Build history of the part. All positions in model axes, mm. Face numbers are marked on the shaded views. A direction names the side the tool comes from. Give positions to 0.01 mm unless a question says otherwise; leave off trailing zeros. Loops run counter-clockwise (first coordinate to the right, second up) from the corner with the lowest first, then second, coordinate; pieces in that order, holes last.
1) Wall check: line 1 (Y direction, x = 38, z = 5.8); line 2 (Z direction, x = 28.5, y = 67); line 3 (Z direction, x = -13, y = 23). Give the ranges that are in metal, low to high.
2) Flat gauge pins, fed straight in: P1, Ø1, axis at x = 73, y = 62, coming from the +Z side; P2, Ø8.5, axis at x = 25, z = 78.88, coming from the +Y side; P3, Ø4.5, axis at x = 18.5, z = 79, coming from the -Y side. Where does each tip first touch, or does it go through?
3) Band-saw the part on B-B on y = 77. List the corners of the cut face in (x, z), then the cut area to 3 significant figures.
4) Band-saw the part on C-C on x = 13.5. List the corners of the cut face in (y, z), then the cut area to 3 significant figures.
5) Band-saw the part on D-D on y = 55. List the corners of the cut face in (x, z), then the cut area to 3 significant figures.
6) Two-plate mould, pull along Y, no slides. Class the marked faces 1, 2 and 3: +Y half, -Y half, draft (parallel to the pull), parting line (faces both ways), or undercut.
7) Band-saw the part on A-A on x = 25. List the corners of the cut face in (y, z).
8) 3-axis set-ups, long thin cutter, end or side, ignore diameter. For the marked faces 4 and 5: which of +Z, -Z, +X, -X, +Y, -Y reach the whole face in a straight line?
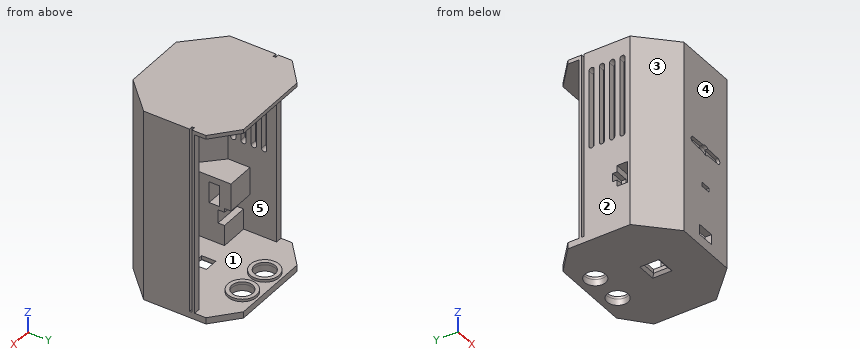
```python
from build123d import *

# Parameters (mm, degrees)
BOSS_EXTRUDE2_DEPTH  = 150
CUT_EXTRUDE2_DEPTH   = 145
CUT_EXTRUDE4_DEPTH   = 145
BOSS_EXTRUDE3_DEPTH  = 90
SKETCH10_W           = 14
SKETCH10_H           = 8
SKETCH10_W_2         = 8.5
SKETCH10_H_2         = 3.2
CUT_EXTRUDE5_DEPTH   = 189.01595677
SKETCH11_W           = 11
SKETCH11_H           = 11
CUT_EXTRUDE6_DEPTH   = 187.413518823
SKETCH12_R           = 11.15
SKETCH12_R_2         = 8.15
BOSS_EXTRUDE4_DEPTH  = 2
SKETCH13_R           = 8.15
CUT_EXTRUDE7_DEPTH   = 187.413518823
CHAMFER1_SIZE        = 2
CUT_EXTRUDE8_REACH   = 166.515
SKETCH14_W           = 45.857864376
SKETCH14_H           = 8
BOSS_EXTRUDE5_REACH  = 179.757
SKETCH15_W           = 22.071067812
SKETCH15_H           = 16.5
BOSS_EXTRUDE6_REACH  = 179.757
SKETCH16_W           = 22.071067812
SKETCH16_H           = 16.5
BOSS_EXTRUDE7_DEPTH  = 22.071067812
BOSS_EXTRUDE9_DEPTH  = 3
SKETCH19_W           = 1
SKETCH19_H           = 2
BOSS_EXTRUDE10_DEPTH = 142
CUT_EXTRUDE9_DEPTH   = 151.203195705
SKETCH21_W           = 16.5
SKETCH21_H           = 8
CUT_EXTRUDE10_DEPTH  = 200.060292374
SKETCH22_W           = 6.5
SKETCH22_H           = 3.5
CUT_EXTRUDE11_DEPTH  = 10
CUT_EXTRUDE13_DEPTH  = 5
CUT_EXTRUDE15_DEPTH  = 2.5
SKETCH28_R           = 3.8
CUT_EXTRUDE16_DEPTH  = 190.15932438
BOSS_EXTRUDE11_DEPTH = 13


with BuildPart() as part:
    # Sketch1 → Boss-Extrude2 (new body)
    with BuildSketch(Plane.XY):
        Polygon((0, 0), (50, 0), (75, 25), (75, 73.483551981), (56, 90), (-6, 90), (-25, 73.483551981), (-25, 25), align=None)
    extrude(amount=BOSS_EXTRUDE2_DEPTH)

    # Sketch3 → Cut-Extrude2 (cut)
    with BuildSketch(Plane.XY.offset(150)):
        Polygon((-4.130576603, 85), (-20, 71.204920704), (-20, 27.071067812), (2.071067812, 5), (47.928932188, 5), (70, 27.071067812), (70, 71.204920704), (54.130576603, 85), align=None)
    extrude(amount=-CUT_EXTRUDE2_DEPTH, mode=Mode.SUBTRACT)

    # Sketch8 → Cut-Extrude4 (cut)
    with BuildSketch(Plane.XY.offset(150)):
        Polygon((-6, 90), (-25, 73.483551981), (-25, 60.75095761), (-22, 60.75095761), (-22, 62.75095761), (-24, 62.75095761), (-24, 64.75095761), (-20, 64.75095761), (-20, 71.204920704), (-4.130576603, 85), (54.130576603, 85), (70, 71.204920704), (70, 64.75095761), (74, 64.75095761), (74, 62.75095761), (72, 62.75095761), (72, 60.75095761), (75, 60.75095761), (75, 73.483551981), (56, 90), align=None)
    extrude(amount=-CUT_EXTRUDE4_DEPTH, mode=Mode.SUBTRACT)

    # Sketch9 → Boss-Extrude3 (add)
    with BuildSketch(Plane.ZY.offset(-70)):
        Polygon((21, 34.071067812), (31.5, 34.071067812), (31.5, 39.071067812), (34.5, 39.071067812), (34.5, 31.071067812), (18, 31.071067812), (18, 39.071067812), (21, 39.071067812), align=None)
    extrude(amount=BOSS_EXTRUDE3_DEPTH)

    # Sketch10 → Cut-Extrude5 (cut, through all)
    with BuildSketch(Plane(origin=(0, 5, 0), x_dir=(1, 0, 0), z_dir=(0, 1, 0))):
        with Locations((25, -12)):
            Rectangle(SKETCH10_W, SKETCH10_H)
        with Locations((25, -49.625084235)):
            Rectangle(SKETCH10_W_2, SKETCH10_H_2)
    extrude(amount=-CUT_EXTRUDE5_DEPTH, mode=Mode.SUBTRACT)

    # Sketch11 → Cut-Extrude6 (cut, through all)
    with BuildSketch(Plane.XY.offset(5)):
        with Locations((25, 38.5)):
            Rectangle(SKETCH11_W, SKETCH11_H)
    extrude(amount=-CUT_EXTRUDE6_DEPTH, mode=Mode.SUBTRACT)

    # Sketch12 → Boss-Extrude4 (add)
    # profile 1 of 2: a face of its own
    with BuildSketch(Plane.XY.offset(5)):
        with Locations(Location((12, 77, 0), (0, 0, 180))):
            Circle(SKETCH12_R)
        with Locations((12, 77)):
            Circle(SKETCH12_R_2, mode=Mode.SUBTRACT)
    # profile 2 of 2: a face of its own
    with BuildSketch(Plane.XY.offset(5)):
        with Locations(Location((38, 77, 0), (0, 0, 180))):
            Circle(SKETCH12_R)
        with Locations((38, 77)):
            Circle(SKETCH12_R_2, mode=Mode.SUBTRACT)
    extrude(amount=BOSS_EXTRUDE4_DEPTH)

    # Sketch13 → Cut-Extrude7 (cut, through all)
    with BuildSketch(Plane.XY.offset(5)):
        with Locations((12, 77)):
            Circle(SKETCH13_R)
        with Locations((38, 77)):
            Circle(SKETCH13_R)
    extrude(amount=-CUT_EXTRUDE7_DEPTH, mode=Mode.SUBTRACT)

    # Chamfer1
    chamfer1_edges = [part.edges().sort_by_distance(p)[0] for p in [
        (19.5, 38.5, 0),
        (25, 44, 0),
        (30.5, 38.5, 0),
        (25, 33, 0),
    ]]
    chamfer(chamfer1_edges, length=CHAMFER1_SIZE)

    # Cut-Extrude8: up to this face of the body (flat: up to its plane)
    cut_extrude8_end = Plane(part.part.faces().sort_by_distance((25, 35.071067812, 18))[0])
    # Sketch14 → Cut-Extrude8 (cut, up to the picked face)
    with BuildSketch(Plane.XY.offset(34.5), mode=Mode.PRIVATE) as cut_extrude8_sk1:
        with Locations((25, 35.071067812)):
            Rectangle(SKETCH14_W, SKETCH14_H)
    cut_extrude8_tool1 = split(extrude(cut_extrude8_sk1.sketch, amount=-CUT_EXTRUDE8_REACH, mode=Mode.PRIVATE), bisect_by=cut_extrude8_end, keep=Keep.BOTH, mode=Mode.PRIVATE)
    add(cut_extrude8_tool1.solids().sort_by(Axis((25, 35.071068, 34.5), (0, 0, -1)))[0], mode=Mode.SUBTRACT)

    # Boss-Extrude5: up to this plane
    boss_extrude5_end = Plane(origin=(47.928932188, 5, -120.415945788), z_dir=(0.7071067811865476, -0.7071067811865475, 0))
    # Sketch15 → Boss-Extrude5 (add, up to the surface)
    with BuildSketch(Plane.XZ.offset(-31.071067812), mode=Mode.PRIVATE) as boss_extrude5_sk1:
        with Locations((58.964466094, 26.25)):
            Rectangle(SKETCH15_W, SKETCH15_H)
    boss_extrude5_tool1 = split(extrude(boss_extrude5_sk1.sketch, amount=BOSS_EXTRUDE5_REACH, mode=Mode.PRIVATE), bisect_by=boss_extrude5_end, keep=Keep.BOTH, mode=Mode.PRIVATE)
    add(boss_extrude5_tool1.solids().sort_by_distance((58.964466, 31.071068, 26.25))[0])

    # Boss-Extrude6: up to this plane
    boss_extrude6_end = Plane(origin=(-20, 27.071067812, -120.415945788), z_dir=(-0.7071067811865475, -0.7071067811865476, 0))
    # Sketch16 → Boss-Extrude6 (add, up to the surface)
    with BuildSketch(Plane.XZ.offset(-31.071067812), mode=Mode.PRIVATE) as boss_extrude6_sk1:
        with Locations((-8.964466094, 26.25)):
            Rectangle(SKETCH16_W, SKETCH16_H)
    boss_extrude6_tool1 = split(extrude(boss_extrude6_sk1.sketch, amount=BOSS_EXTRUDE6_REACH, mode=Mode.PRIVATE), bisect_by=boss_extrude6_end, keep=Keep.BOTH, mode=Mode.PRIVATE)
    add(boss_extrude6_tool1.solids().sort_by_distance((-8.964466, 31.071068, 26.25))[0])

    # Sketch17 → Boss-Extrude7 (add)
    with BuildSketch(Plane(origin=(-20, 0, 0), x_dir=(0, 0, -1), z_dir=(1, 0, 0))):
        Polygon((-56, 27.071067812), (-51, 27.071067812), (-51, 35.071067812), (-34.5, 35.071067812), (-34.5, 39.071067812), (-34.5, 44.071067812), (-56, 44.071067812), align=None)
        Polygon((-34.5, 5), (-34.5, 27.071067812), (-51, 27.071067812), (-56, 27.071067812), (-56, 5), align=None)
    extrude(amount=BOSS_EXTRUDE7_DEPTH)

    # Sketch18 → Boss-Extrude9 (add)
    with BuildSketch(Plane.XY.offset(150)):
        Polygon((75, 62.75095761), (75, 73.483551981), (56, 90), (-6, 90), (-25, 73.483551981), (-25, 62.75095761), (-24, 62.75095761), (-24, 64.75095761), (-20, 64.75095761), (-20, 27.071067812), (2.071067812, 5), (47.928932188, 5), (70, 27.071067812), (70, 64.75095761), (74, 64.75095761), (74, 62.75095761), align=None)
    extrude(amount=-BOSS_EXTRUDE9_DEPTH)

    # Sketch19 → Boss-Extrude10 (add)
    with BuildSketch(Plane(origin=(0, 0, 147), x_dir=(-1, 0, 0), z_dir=(0, 0, -1))):
        with Locations((-74.5, 63.75095761)):
            Rectangle(SKETCH19_W, SKETCH19_H)
        with Locations((24.5, 63.75095761)):
            Rectangle(SKETCH19_W, SKETCH19_H)
    extrude(amount=BOSS_EXTRUDE10_DEPTH)

    # Sketch20 → Cut-Extrude9 (cut, through all)
    with BuildSketch(Plane.XY.offset(56)):
        Polygon((-5, 5), (-20, 20), (-20, 5), align=None)
    extrude(amount=-CUT_EXTRUDE9_DEPTH, mode=Mode.SUBTRACT)

    # Sketch21 → Cut-Extrude10 (cut, through all)
    with BuildSketch(Plane(origin=(-20, 0, 0), x_dir=(0, 0, -1), z_dir=(1, 0, 0))):
        with Locations((-42.75, 31.071067812)):
            Rectangle(SKETCH21_W, SKETCH21_H)
    extrude(amount=-CUT_EXTRUDE10_DEPTH, mode=Mode.SUBTRACT)

    # Sketch22 → Cut-Extrude11 (cut)
    with BuildSketch(Plane.ZY.offset(25)):
        with Locations((42.75, 36.821067812)):
            Rectangle(SKETCH22_W, SKETCH22_H)
    extrude(amount=-CUT_EXTRUDE11_DEPTH, mode=Mode.SUBTRACT)

    # Sketch23 → Cut-Extrude13 (cut)
    with BuildSketch(Plane.ZY.offset(25)):
        with BuildLine():
            Line((75, 29), (135, 29))
            ThreePointArc((135, 29), (137, 31), (135, 33))
            Line((135, 33), (75, 33))
            ThreePointArc((75, 33), (73, 31), (75, 29))
        make_face()
        with BuildLine():
            Line((135, 41), (75, 41))
            ThreePointArc((75, 41), (73, 39), (75, 37))
            Line((75, 37), (135, 37))
            ThreePointArc((135, 37), (137, 39), (135, 41))
        make_face()
        with BuildLine():
            Line((135, 49), (75, 49))
            ThreePointArc((75, 49), (73, 47), (75, 45))
            Line((75, 45), (135, 45))
            ThreePointArc((135, 45), (137, 47), (135, 49))
        make_face()
        with BuildLine():
            Line((135, 57), (75, 57))
            ThreePointArc((75, 57), (73, 55), (75, 53))
            Line((75, 53), (135, 53))
            ThreePointArc((135, 53), (137, 55), (135, 57))
        make_face()
    extrude(amount=-CUT_EXTRUDE13_DEPTH, mode=Mode.SUBTRACT)

    # Sketch27 → Cut-Extrude15 (cut)
    with BuildSketch(Plane.XZ):
        with BuildLine():
            Line((39.404762454, 81.167250077), (39.404762454, 81.166207685))
            ThreePointArc((39.404762454, 81.166207685), (41.672056129, 78.884218387), (39.404762454, 76.60222909))
            Line((39.404762454, 76.60222909), (39.404762454, 76.601183426))
            Line((39.404762454, 76.601183426), (27.659446006, 76.169652537))
            ThreePointArc((27.659446006, 76.169652537), (25.117179913, 75.085745409), (22.512932044, 76.010874907))
            Line((22.512932044, 76.010874907), (10.566254086, 76.601183426))
            ThreePointArc((10.566254086, 76.601183426), (8.393884355, 78.898098023), (10.595237546, 81.167250077))
            Line((10.595237546, 81.167250077), (22.340553994, 81.598223966))
            ThreePointArc((22.340553994, 81.598223966), (25, 82.683938251), (27.659446006, 81.598223966))
            Line((27.659446006, 81.598223966), (39.404762454, 81.167250077))
        make_face()
    extrude(amount=-CUT_EXTRUDE15_DEPTH, mode=Mode.SUBTRACT)

    # Sketch28 → Cut-Extrude16 (cut, through all)
    with BuildSketch(Plane.XZ.offset(-2.5)):
        with Locations(Location((25, 78.883938251, 0), (0, 0, 45.584691403))):
            Circle(SKETCH28_R)
    extrude(amount=-CUT_EXTRUDE16_DEPTH, mode=Mode.SUBTRACT)

    # Sketch29 → Boss-Extrude11 (add)
    with BuildSketch(Plane(origin=(0, 0, 18), x_dir=(-1, 0, 0), z_dir=(0, 0, -1))):
        Polygon((-70, 39.071067812), (-70, 27.071067812), (-47.928932188, 5), (-47.928932188, 39.071067812), align=None)
        Polygon((20, 39.071067812), (-2.071067812, 39.071067812), (-2.071067812, 5), (20, 27.071067812), align=None)
    extrude(amount=BOSS_EXTRUDE11_DEPTH)


solid = part.part
```
Findings below:
1. line 1: y = 0 to 5, 65.85 to 68.85, 85.15 to 88.15
1. line 2: z = 0 to 5, 147 to 150
1. line 3: z = 0 to 56, 147 to 150
2. P1: stops at z = 5
2. P2: stops at y = 5
2. P3: stops at y = 2.5
3. outline: (-20.95, 0) - (3.85, 0) - (3.85, 7) - (0.85, 7) - (0.85, 5) - (-20.95, 5) - close; (-20.95, 147) - (70.95, 147) - (70.95, 150) - (-20.95, 150) - close; (20.15, 0) - (29.85, 0) - (29.85, 7) - (26.85, 7) - (26.85, 5) - (23.15, 5) - (23.15, 7) - (20.15, 7) - close; (46.15, 0) - (70.95, 0) - (70.95, 5) - (49.15, 5) - (49.15, 7) - (46.15, 7) - close
3. area: 596 mm2
4. outline: (0, 0) - (68.99, 0) - (68.99, 7) - (65.95, 7) - (65.95, 5) - (5, 5) - (5, 147) - (90, 147) - (90, 150) - (0, 150) - (0, 81.27) - (2.5, 81.27) - (2.5, 76.46) - (0, 76.46) - close; (85.01, 0) - (90, 0) - (90, 5) - (88.05, 5) - (88.05, 7) - (85.01, 7) - close
4. area: 1,350 mm2
5. outline: (-25, 0) - (75, 0) - (75, 150) - (-25, 150) - (-25, 137) - (-20, 137) - (-20, 147) - (70, 147) - (70, 5) - (-20, 5) - (-20, 73) - (-25, 73) - close
5. area: 1,900 mm2
6. face 1: undercut
6. face 2: draft
6. face 3: -Y half
7. outline: (0, 0) - (31, 0) - (33, 2) - (33, 5) - (5, 5) - (5, 8) - (0, 8) - close; (0, 16) - (5, 16) - (5, 48.03) - (0, 48.03) - close; (0, 51.23) - (5, 51.23) - (5, 75.08) - (0, 75.08) - close; (0, 82.68) - (5, 82.68) - (5, 147) - (90, 147) - (90, 150) - (0, 150) - close; (44, 2) - (46, 0) - (90, 0) - (90, 5) - (44, 5) - close
8. face 4: +Z, -Z, +X, -X, -Y
8. face 5: +Y
